```python
from build123d import *

# Parameters (mm, degrees)
F1_DEPTH = 25.4


with BuildPart() as f1:
    # F0 (on Top) → F1 (new body)
    with BuildSketch(Plane.XY):
        Polygon((-9.9282488227, 16.6444163769), (-9.9282488227, -38.8369709253), (-6.8141991987, -38.8369709253), (-4.3801111169, -38.8369709253), (-1.1680317111, -38.8369709253), (3.4067514008, -38.8369709253), (6.1321551912, -38.8369709253), (8.7602203712, -38.8369709253), (8.7602203712, 16.6444163769), (0, 16.6444163769), (-3.5040895455, 16.6444163769), (-6.8141991987, 16.6444163769), align=None)
        Polygon((-20.4405128956, 23.6525926739), (-9.9282488227, 16.6444163769), (-6.8141991987, 16.6444163769), (-12.2392783805, 23.6525926739), (-12.264306657, 23.6525926739), align=None)
        Polygon((-39.7129952908, 23.6525926739), (-9.9282488227, 16.6444163769), (-20.4405128956, 23.6525926739), align=None)
        Polygon((-12.2392783805, 23.6525926739), (-6.8141991987, 16.6444163769), (-3.5040895455, 16.6444163769), (-6.6358093424, 39.7052673339), (0, 27.0106745884), (0, 40.0465349111), (0, 51.3932853937), (-6.2433463768, 67.9810519437), (-16.1107429013, 68.2416611761), (-23.2746789764, 63.9495998621), (-15.1843791828, 53.4984625885), (-21.9592093912, 36.2089052796), (-18.098320559, 31.2213670903), align=None)
        Polygon((-6.8141991987, 47.2179802464), (-7.5501442092, 46.4380983203), (-9.9282488227, 63.9495998621), align=None, mode=Mode.SUBTRACT)
        Polygon((-30.4814127266, 30.3465261318), (-20.4405128956, 23.6525926739), (-12.264306657, 23.6525926739), (-12.2392783805, 23.6525926739), (-18.098320559, 31.2213670903), (-30.4814127266, 32.9626211831), align=None)
        Polygon((-39.7129952908, 23.6525926739), (-20.4405128956, 23.6525926739), (-30.4814127266, 30.3465261318), (-30.4814127266, 32.9626211831), (-45.2611297369, 35.0408777595), align=None)
        Polygon((3.4067514008, -38.8369709253), (-1.1680317111, -38.8369709253), (-1.1680317111, -59.2774823308), align=None)
        Polygon((-6.6358093424, 39.7052673339), (-3.5040895455, 16.6444163769), (0, 16.6444163769), (0, 21.9005476683), (0, 27.0106745884), align=None)
        Polygon((-49.3492335081, 51.3932853937), (-45.2611297369, 35.0408777595), (-30.4814127266, 32.9626211831), (-18.098320559, 31.2213670903), (-21.9592093912, 36.2089052796), (-30.4814127266, 47.2179802464), align=None)
        Polygon((0, 21.9005476683), (0, 16.6444163769), (8.7602203712, 16.6444163769), (15.9789933035, 43.8407290326), (18.5424652882, 53.4984625885), (21.3165320456, 63.9495998621), (34.1648571193, 70.665769279), (13.7243429199, 67.4536824226), (0, 56.9414235651), (0, 51.3932853937), (0, 40.0465349111), (0, 27.0106745884), align=None)
        Polygon((-41.173029691, 61.0295273364), (-49.3492335081, 51.3932853937), (-30.4814127266, 47.2179802464), (-33.7135461765, 51.3932853937), align=None)
        Polygon((8.7602203712, -38.8369709253), (6.1321551912, -38.8369709253), (8.7602203712, -59.2774823308), align=None)
        Polygon((15.9789933035, 43.8407290326), (8.7602203712, 16.6444163769), (18.5424652882, 27.0106745884), (28.3247102052, 37.3769327998), (38.2691381014, 47.9150565343), (48.2135659976, 58.4531802689), (34.1648571193, 70.665769279), (21.3165320456, 63.9495998621), (18.5424652882, 53.4984625885), align=None)
        Polygon((18.5424652882, 27.0106745884), (8.7602203712, 16.6444163769), (40.5890159309, 21.9005476683), (49.3492297828, 58.1094510853), (28.3247102052, 37.3769327998), align=None)
        Polygon((-30.4814127266, 47.2179802464), (-21.9592093912, 36.2089052796), (-15.1843791828, 53.4984625885), (-23.2746789764, 63.9495998621), (-16.1107429013, 68.2416611761), (-30.4322889094, 68.6199095927), (-33.7135461765, 51.3932853937), align=None)
        Polygon((-30.4322889094, 68.6199095927), (-41.173029691, 61.0295273364), (-33.7135461765, 51.3932853937), align=None)
        Polygon((-6.2433463768, 67.9810519437), (0, 51.3932853937), (0, 56.9414235651), (0, 67.8161580224), align=None)
        Polygon((0, 67.8161580224), (0, 56.9414235651), (13.7243429199, 67.4536824226), align=None)
    extrude(amount=F1_DEPTH)


solid = f1.part
```
Input: part model. Units: mm. Frame: model coordinates. A direction names the side the tool comes from. Coordinates: 2 decimals unless noted, no trailing zeros. Write each loop counter-clockwise with the first axis right and the second up, starting at its lowest first coordinate (ties: lowest second). Pieces come first, ordered by that corner, then holes. Notation, with made-up numbers: (-38, 29) -> (5, 29) arc R30 cw to (5, 64) -> close; hole circle Ø9 at (66.5, 86.5). An arc over 180 degrees is marked (long way). Write each question's results on one line, items separated by ' | '.
Item 1: Material intervals for probe 1 along X at (y, z) = (54, 22.25) (3 decimals); probe 2 along Y at (x, z) = (37, 5.75); probe 3 along X at (y, z) = (-21.5, 16.5), sorted ascending.
Conclusion:
probe 1: x = -47.137 to -8.577, -8.076 to 44.011, 45.182 to 48.355 | probe 2: y = 21.31 to 45.93, 46.57 to 68.2 | probe 3: x = -9.93 to 8.76
Item 2: Pin query (flat end, axial travel): pin 1 Ø10 at (y, z) = (39.5, 18.5) entering from +X; pin 2 Ø6 at (y, z) = (-54, 18) entering from -X; pin 3 Ø5 at (y, z) = (55.5, 4) entering from +X; pin 4 Ø3 at (x, y) = (-13.5, 14.5) entering from +Z. Return the tip coordinate at first contact, or that it passes through.
Conclusion:
pin 1: stops at x = 46.06 | pin 2: stops at x = -1.17 | pin 3: stops at x = 49.32 | pin 4: passes through
Item 3: Section query B-B on y = -46. Return loops of the section in (x, z).
Conclusion:
outline: (-1.17, 0) -> (1.8, 0) -> (1.8, 25.4) -> (-1.17, 25.4) -> close; (7.05, 0) -> (8.76, 0) -> (8.76, 25.4) -> (7.05, 25.4) -> close
Item 4: Mould query, pull axis Y, two halves, no side actions, for faces 6 (the flat face through (-8.723, 55.071, 12.522)), 7 (the flat face through (1.087, -49.2, 12.522)), 8 (the flat face through (-35.727, 64.878, 12.522)). Classes: +Y half, -Y half, draft (parallel to the pull), parting line (faces both ways), or undercut.
Conclusion:
face 6: undercut | face 7: -Y half | face 8: +Y half
Item 5: Set-up query: faces 1 (the flat face through (-1.168, -49, 13)), 2 (the flat face through (5, -38.837, 13)), 3 (the flat face through (24.088, 69.082, 12.522)), 4 (the flat face through (8.76, -22, 13)), 5 (the flat face through (41.29, 64.47, 12.52)). Return all of +Z, -Z, +X, -X, +Y, -Y with unobstructed straight access to the full face (end or side cutting, diameter ignored); none if empty.
Conclusion:
face 1: +Z, -Z, -X, -Y | face 2: +Z, -Z, -Y | face 3: +Z, -Z, +Y | face 4: +Z, -Z, +X, -Y | face 5: +Z, -Z, +X, +Y
Item 6: Section query A-A on z = 3. Return loops of the section in (x, y), plus the area to 3 significant figures.
Conclusion:
outline: (-49.35, 51.39) -> (-45.26, 35.04) -> (-39.71, 23.65) -> (-9.93, 16.64) -> (-9.93, -38.84) -> (-1.17, -38.84) -> (-1.17, -59.28) -> (3.41, -38.84) -> (6.13, -38.84) -> (8.76, -59.28) -> (8.76, 16.64) -> (40.59, 21.9) -> (49.35, 58.11) -> (28.32, 37.38) -> (48.21, 58.45) -> (34.16, 70.67) -> (13.72, 67.45) -> (-30.43, 68.62) -> (-41.17, 61.03) -> close; hole (-9.93, 63.95) -> (-7.55, 46.44) -> (-6.81, 47.22) -> close | area: 5,420 mm^2
Item 7: Section query C-C on y = -26. Return loops of the section in (x, z), plus the area to 3 significant figures.
Conclusion:
outline: (-9.93, 0) -> (8.76, 0) -> (8.76, 25.4) -> (-9.93, 25.4) -> close | area: 475 mm^2
Item 8: Section query D-D on x = 10.5. Return loops of the section in (y, z).
Conclusion:
outline: (16.93, 0) -> (67.54, 0) -> (67.54, 25.4) -> (16.93, 25.4) -> close
